Check sheet for the drawn part. Datum: minimum x, y, z corner. Units: mm. Round coordinates to 2 decimals unless told otherwise and drop trailing zeros. Write each loop counter-clockwise with the first axis right and the second up, starting at its lowest first coordinate (ties: lowest second). Pieces come first, ordered by that corner, then holes. Notation, with made-up numbers: (-5, 79.5) -> (33, 79.5) arc R27 ccw to (33, 97.5) -> close; hole circle Ø6 at (3.5, 51). An arc over 180 degrees is marked (long way). Use CSV: the item, a comma, the result in double quotes.
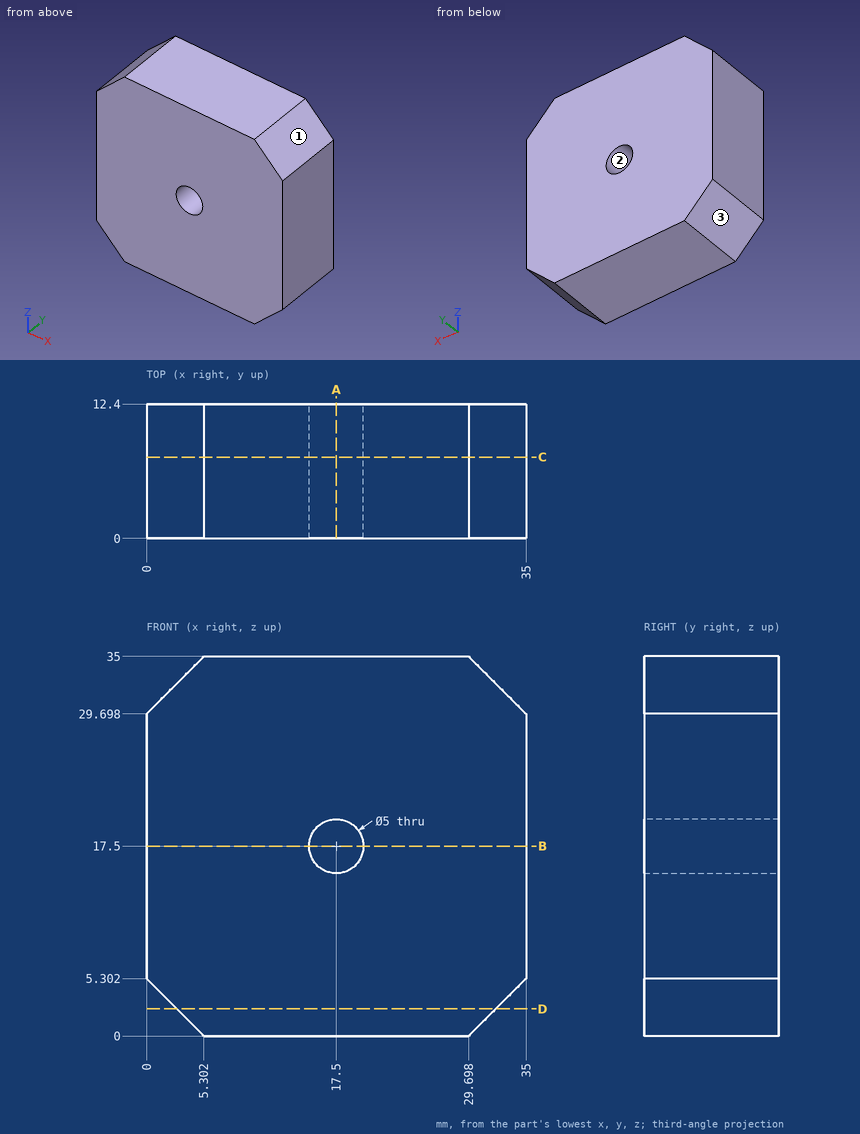
Q1. Material ranges on L1, parallel to X at y = 4, z = 17.5; L2, parallel to Z at x = 31.5, y = 4.75; L3, parallel to Z at x = 15.5, y = 8.75, recorded low to high.
Filled in:
L1,"0 to 15, 20 to 35"
L2,"1.8 to 33.2"
L3,"0 to 16, 19 to 35"
Q2. Go/stop test with a flat-tipped pin: P1, Ø2, axis at x = 19.5, y = 7.5, coming from the -Z side. Record where the tip stops, or that it passes through.
Filled in:
P1,"z = 0"
Q3. Section check D-D (z = 2.5). Record the cut outline in (x, y).
Filled in:
outline,"(2.8, 0) -> (32.2, 0) -> (32.2, 12.4) -> (2.8, 12.4) -> close"
Q4. Section check B-B (z = 17.5). Record the cut outline in (x, y), plus the area to 3 significant figures.
Filled in:
outline,"(0, 0) -> (15, 0) -> (15, 12.4) -> (0, 12.4) -> close; (20, 0) -> (35, 0) -> (35, 12.4) -> (20, 12.4) -> close"
area,"372 mm²"
Q5. Mould release check, pull along X, two halves, no side actions. Record for the marked faces 1, 2 and 3: released by +X, released by -X, zero draft, split by the parting line, or undercut.
Filled in:
face 1,"released by +X"
face 2,"undercut"
face 3,"released by -X"
Q6. Section check A-A (x = 17.5). Record the cut outline in (y, z).
Filled in:
outline,"(0, 0) -> (12.4, 0) -> (12.4, 15) -> (0, 15) -> close; (0, 20) -> (12.4, 20) -> (12.4, 35) -> (0, 35) -> close"
Q7. Section check C-C (y = 7.5). Record the cut outline in (x, z), plus the area to 3 significant figures.
Filled in:
outline,"(0, 5.3) -> (5.3, 0) -> (29.7, 0) -> (35, 5.3) -> (35, 29.7) -> (29.7, 35) -> (5.3, 35) -> (0, 29.7) -> close; hole circle Ø5 at (17.5, 17.5)"
area,"1,150 mm²"
